Geometry: final body of the model. Coordinates: model frame, mm. A direction names the side the tool comes from. Coordinates: 2 decimals unless noted, no trailing zeros. Loops run counter-clockwise (first coordinate to the right, second up) from the corner with the lowest first, then second, coordinate; pieces in that order, holes last. Notation, with made-up numbers: (73, 66.25) - (78, 66.25) arc R19 ccw to (78, 83.25) - close; hole circle Ø1 at (50.25, 71.5). An arc over 180 degrees is marked (long way). Return JSON: item names as keys, results as strings.
from build123d import *

# Parameters (mm, degrees)
SKETCH2_R           = 16.7
SKETCH2_R_2         = 12.85
BOSS_EXTRUDE1_DEPTH = 100
SKETCH3_R           = 16.7
BOSS_EXTRUDE2_DEPTH = 5
SKETCH4_R           = 16.7
SKETCH4_R_2         = 5
BOSS_EXTRUDE3_DEPTH = 5


with BuildPart() as part:
    # Sketch2 → Boss-Extrude1 (new body)
    with BuildSketch(Plane.XY):
        Circle(SKETCH2_R)
        Circle(SKETCH2_R_2, mode=Mode.SUBTRACT)
    extrude(amount=BOSS_EXTRUDE1_DEPTH)

    # Sketch3 → Boss-Extrude2 (add)
    with BuildSketch(Plane(origin=(0, 0, 0), x_dir=(-1, 0, 0), z_dir=(0, 0, -1))):
        Circle(SKETCH3_R)
    extrude(amount=BOSS_EXTRUDE2_DEPTH)

    # Sketch4 → Boss-Extrude3 (add)
    with BuildSketch(Plane.XY.offset(100)):
        Circle(SKETCH4_R)
        Circle(SKETCH4_R_2, mode=Mode.SUBTRACT)
    extrude(amount=BOSS_EXTRUDE3_DEPTH)


solid = part.part
Item 1: Section query D-D, the plane z = 89. Return loops of the section in (x, y).
Worked out:
{"outline": "circle Ø33.4 at (0, 0); hole circle Ø25.7 at (0, 0)"}
Item 2: Mould query, pull axis X, two halves, no side actions, for faces 1 (the face through (0, 0, 0)), 2 (the face through (0, 0, -5)). Classes: +X half, -X half, draft (parallel to the pull), parting line (faces both ways), or undercut.
Worked out:
{"face 1": "undercut", "face 2": "draft"}
Item 3: Ray query, probe 1 along Z at (x, y) = (3.5, 9.5); probe 2 along Y at (x, z) = (0, 33); probe 3 along Y at (x, z) = (3, 16.5). Return the intervals inside material, ascending. Write a range as from..to.
Worked out:
{"probe 1": "-5..0, 100..105", "probe 2": "-16.7..-12.85, 12.85..16.7", "probe 3": "-16.43..-12.49, 12.49..16.43"}
Item 4: First-contact query: pin 1 Ø1.5 at (x, z) = (8.5, 33) entering from +Y; pin 2 Ø6 at (x, y) = (0, 0) entering from +Z; pin 3 Ø12 at (x, z) = (6, 27.5) entering from -Y; pin 4 Ø1 at (y, z) = (-8, 33) entering from +X. Flat tips, straight axial feed; report the tip coordinate or a pass-through.
Worked out:
{"pin 1": "y = 14.79", "pin 2": "z = 0", "pin 3": "y = -16.7", "pin 4": "x = 14.92"}
Item 5: Reachability of faces 3 (the face through (-3.9, -3.5, 105)), 4 (the face through (-1.08, -4.88, 102.46)), 5 (the face through (-10.197, -7.819, 49.3)) from +Z, -Z, +X, -X, +Y, -Y: full face, straight path, thin tool, end or side. Return the list, or none.
Worked out:
{"face 3": "+Z, +X, -X, +Y, -Y", "face 4": "+Z", "face 5": "none"}
Item 6: Section query A-A, the plane y = 8.5. Return loops of the section in (x, z), and give its area (3 significant figures).
Worked out:
{"outline": "(-14.37, -5) - (14.37, -5) - (14.37, 105) - (-14.37, 105) - close; hole (-9.64, 0) - (9.64, 0) - (9.64, 100) - (-9.64, 100) - close", "area": "1,240 mm^2"}
Item 7: Section query B-B, the plane x = 0. Return loops of the section in (y, z), and give its area (3 significant figures).
Worked out:
{"outline": "(-16.7, -5) - (16.7, -5) - (16.7, 105) - (5, 105) - (5, 100) - (12.85, 100) - (12.85, 0) - (-12.85, 0) - (-12.85, 100) - (-5, 100) - (-5, 105) - (-16.7, 105) - close", "area": "1,050 mm^2"}
